Geometry: see drawing. Coordinates: mm, zero at the bounding-box minimum. Coordinates: 2 decimals unless noted, no trailing zeros. Loops run counter-clockwise (first coordinate to the right, second up) from the corner with the lowest first, then second, coordinate; pieces in that order, holes last. Notation, with made-up numbers: (53, 50.25) -> (71, 50.25) arc R18 cw to (71, 62.25) -> close; hole circle Ø4 at (-2.5, -1.5). An arc over 180 degrees is marked (long way). One line per item, written item: value. Start each with the question number.
Item 1: Ray query, probe 1 along Z at (x, y) = (0.95, 1.5); probe 2 along Z at (x, y) = (0.75, 6.75); probe 3 along Y at (x, z) = (0.4, 14). Return the intervals inside material, ascending. Write a range as from..to.
Item 2: Contact query for flat-ended pins moving along their axis: pin 1 Ø1.3 at (y, z) = (19.5, 1.5) entering from -X; pin 2 Ø1.8 at (y, z) = (19.5, 23.5) entering from -X. Output: stop coordinate, or through.
Item 3: Section query C-C on x = 0.2. Return loops of the section in (y, z).
Item 4: Section query A-A on y = 11.25. Return loops of the section in (x, z).
Item 5: Section query D-D on z = 12.75. Return loops of the section in (x, y), then the cut area to 3 significant figures.
Item 6: Section query B-B on z = 23.5. Return loops of the section in (x, y), then the cut area to 3 significant figures.
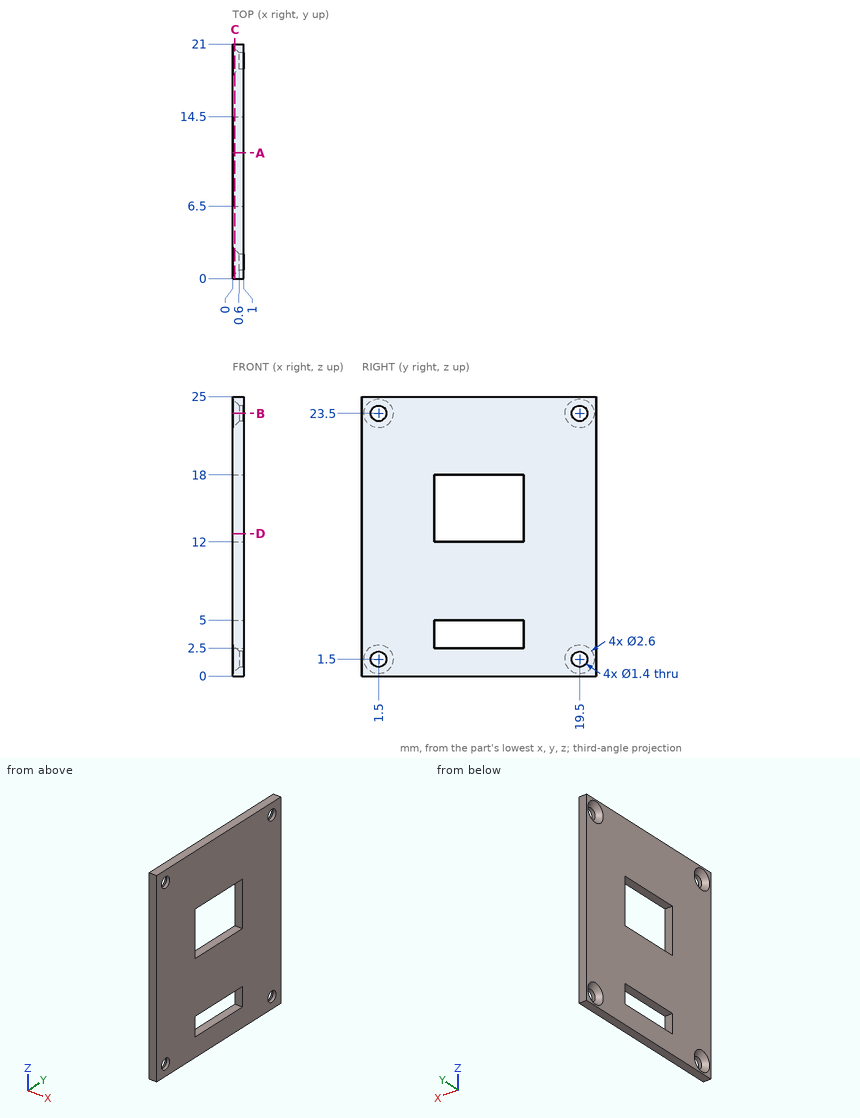
Reply:
1. probe 1: z = 0..0.8, 2.2..22.8, 24.2..25
1. probe 2: z = 0..2.5, 5..12, 18..25
1. probe 3: y = 0..6.5, 14.5..21
2. pin 1: passes through
2. pin 2: stops at x = 0.4
3. outline: (0, 0) -> (21, 0) -> (21, 25) -> (0, 25) -> close; hole circle Ø2.2 at (1.5, 1.5); hole circle Ø2.2 at (1.5, 23.5); hole (6.5, 2.5) -> (14.5, 2.5) -> (14.5, 5) -> (6.5, 5) -> close; hole (6.5, 12) -> (14.5, 12) -> (14.5, 18) -> (6.5, 18) -> close; hole circle Ø2.2 at (19.5, 1.5); hole circle Ø2.2 at (19.5, 23.5)
4. outline: (0, 0) -> (1, 0) -> (1, 2.5) -> (0, 2.5) -> close; (0, 5) -> (1, 5) -> (1, 12) -> (0, 12) -> close; (0, 18) -> (1, 18) -> (1, 25) -> (0, 25) -> close
5. outline: (0, 0) -> (1, 0) -> (1, 6.5) -> (0, 6.5) -> close; (0, 14.5) -> (1, 14.5) -> (1, 21) -> (0, 21) -> close
5. area: 13.0 mm²
6. outline: (0, 0) -> (1, 0) -> (1, 0.8) -> (0.6, 0.8) -> (0, 0.2) -> close; (0, 2.8) -> (0.6, 2.2) -> (1, 2.2) -> (1, 18.8) -> (0.6, 18.8) -> (0, 18.2) -> close; (0, 20.8) -> (0.6, 20.2) -> (1, 20.2) -> (1, 21) -> (0, 21) -> close
6. area: 17.5 mm²
